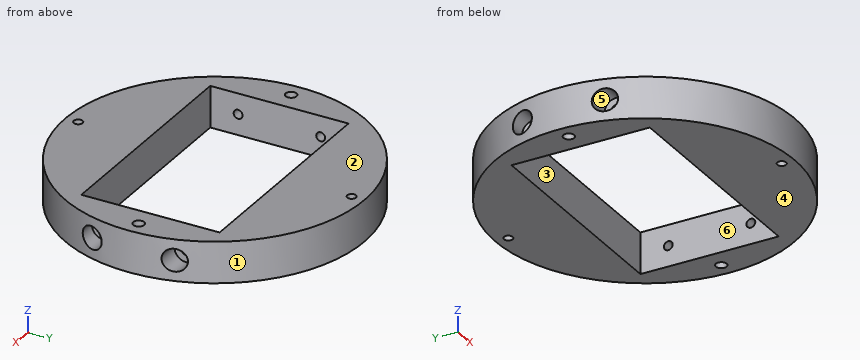
from build123d import *

# Parameters (mm, degrees)
EXTRUDE_2_OUTLINE_R      = 72.5
EXTRUDE_2_OUTLINE_R_2    = 2.15
EXTRUDE_2_OUTLINE_R_3    = 2.65
EXTRUDE_2_OUTLINE_W      = 110
EXTRUDE_2_OUTLINE_H      = 67
EXTRUDE_2_DEPTH          = 20
CUT_EXTRUDE_2_DEPTH      = 149.028713431
CUT_EXTRUDE_2_DEPTH_BACK = 149.028713431
SKETCH_5_R               = 2.15
SKETCH_6_R               = 5.5
CUT_EXTRUDE_4_DEPTH      = 153.35649


# Read off the part's stored shape, not the designer's step: the extrude step
with BuildPart() as part:
    # Extrude 2 outline → Extrude 2 (new body)
    with BuildSketch(Plane.XY):
        Circle(EXTRUDE_2_OUTLINE_R)
        with Locations((0, -66.25)):
            Circle(EXTRUDE_2_OUTLINE_R_2, mode=Mode.SUBTRACT)
        with Locations((-65, 0)):
            Circle(EXTRUDE_2_OUTLINE_R_3, mode=Mode.SUBTRACT)
        Rectangle(EXTRUDE_2_OUTLINE_W, EXTRUDE_2_OUTLINE_H, mode=Mode.SUBTRACT)
        with Locations((65, 0)):
            Circle(EXTRUDE_2_OUTLINE_R_3, mode=Mode.SUBTRACT)
        with Locations((0, 66.25)):
            Circle(EXTRUDE_2_OUTLINE_R_2, mode=Mode.SUBTRACT)
    extrude(amount=EXTRUDE_2_DEPTH)

    # Sketch 5 → Cut-Extrude 2 (cut, two sides: drawn at the far end of the back side and taken through both)
    with BuildSketch(Plane(origin=(-55, 0, 0), x_dir=(0, 0, -1), z_dir=(1, 0, 0)).offset(-CUT_EXTRUDE_2_DEPTH_BACK)):
        with Locations((-10, 20)):
            Circle(SKETCH_5_R)
        with Locations((-10, -20)):
            Circle(SKETCH_5_R)
    extrude(amount=CUT_EXTRUDE_2_DEPTH + CUT_EXTRUDE_2_DEPTH_BACK, mode=Mode.SUBTRACT)

    # Sketch 6 → Cut-Extrude 4 (cut, through all)
    with BuildSketch(Plane(origin=(60, 0, 0), x_dir=(0, 0, -1), z_dir=(1, 0, 0))):
        with Locations(Location((-10, 20, 0), (0, 0, 180))):
            Circle(SKETCH_6_R)
        with Locations(Location((-10, -20, 0), (0, 0, 180))):
            Circle(SKETCH_6_R)
    cut_extrude_4 = extrude(amount=CUT_EXTRUDE_4_DEPTH, mode=Mode.SUBTRACT)

    # Mirror 1: Cut-Extrude 4 across plane
    add(cut_extrude_4.mirror(Plane(origin=(0, 0, 0), x_dir=(0, 0, 1), z_dir=(1, 0, 0))), mode=Mode.SUBTRACT)


solid = part.part
Work out the finished part from the listing and answer in its coordinate system (mm). Face numbers are marked on the shaded views. A direction names the side the tool comes from. Round coordinates to 2 decimals unless told otherwise and drop trailing zeros. Write each loop counter-clockwise with the first axis right and the second up, starting at its lowest first coordinate (ties: lowest second). Pieces come first, ordered by that corner, then holes. Notation, with made-up numbers: (76, 5) -> (100, 5) arc R14 cw to (100, 25) -> close; hole circle Ø4 at (47, -4.75). An arc over 180 degrees is marked (long way). Answer as CSV lines item,"result". Start each with the question number.
(1) The part is cut by section A-A, the plane x = 0. Give the vertices of the cut face in (y, z), then the cut area to 3 significant figures.
(2) The part is cut by section B-B, the plane x = 65. Give the vertices of the cut face in (y, z).
(3) The part is cut by section D-D, the plane z = 10.5. Give the number of separate pieces and of enclosed holes in the cut face, then the cut area to 3 significant figures.
(4) The part is cut by section C-C, the plane y = -66.25. Give the vertices of the cut face in (x, z).
(5) Each of these flat-tipped pins is pushed along its axis until it touches: pin 1 (12 mm diameter, centred on x = 45, z = 8.5, fed in from -Y); pin 2 (2 mm diameter, centred on y = 50, z = 12.5, fed in from +X); pin 3 (10 mm diameter, centred on x = 9, z = 5.5, fed in from +Y). Where does it stop, or does it pass through?
(6) Find the intervals of material crossed by probe 1 along Y at (x, z) = (0, 10); probe 2 along Z at (x, y) = (56, 20); probe 3 along Y at (x, z) = (56.7, 10), in increasing order.
(7) The mould has two halves that part along Y. Classify the marked faces 1, 2 and 3: +Y half, -Y half, draft (parallel to the pull), parting line (faces both ways), or undercut.
(8) A tool of negligible diameter and unlimited length cuts with its end or side. For the marked faces 4, 5 and 6, from which of +Z, -Z, +X, -X, +Y, -Y can it reach the whole face along a straight path? Write none if from no direction.
Output values:
1,outline,"(-72.5, 0) -> (-68.4, 0) -> (-68.4, 20) -> (-72.5, 20) -> close; (-64.1, 0) -> (-33.5, 0) -> (-33.5, 20) -> (-64.1, 20) -> close; (33.5, 0) -> (64.1, 0) -> (64.1, 20) -> (33.5, 20) -> close; (68.4, 0) -> (72.5, 0) -> (72.5, 20) -> (68.4, 20) -> close"
1,area,"1,390 mm²"
2,outline,"(-32.11, 0) -> (-2.65, 0) -> (-2.65, 20) -> (-32.11, 20) -> close; (2.65, 0) -> (32.11, 0) -> (32.11, 20) -> (2.65, 20) -> close; hole circle Ø11 at (-20, 10); hole circle Ø11 at (20, 10)"
3,separate pieces,"4"
3,enclosed holes,"4"
3,area,"8,570 mm²"
4,outline,"(-29.45, 0) -> (-2.15, 0) -> (-2.15, 20) -> (-29.45, 20) -> close; (2.15, 0) -> (29.45, 0) -> (29.45, 20) -> (2.15, 20) -> close"
5,pin 1,"stops at y = -61.12"
5,pin 2,"stops at x = 53.43"
5,pin 3,"stops at y = 72.39"
6,probe 1,"y = -72.5 to -68.4, -64.1 to -33.5, 33.5 to 64.1, 68.4 to 72.5"
6,probe 2,"z = 0 to 7.85, 12.15 to 20"
6,probe 3,"y = -45.18 to -22.15, -17.85 to 17.85, 22.15 to 45.18"
7,face 1,"parting line"
7,face 2,"draft"
7,face 3,"undercut"
8,face 4,"-Z, +X, -X, +Y, -Y"
8,face 5,"-X"
8,face 6,"+Z, -Z"
